```python
from build123d import *

# Parameters (mm, degrees)
EXTRUDE_1_DEPTH              = 10
SKETCH_2_W                   = 43
SKETCH_2_H                   = 10
EXTRUDE_2_DEPTH              = 24.24999999999997
EXTRUDE_3_DEPTH              = 6.6999999999999975
CUT_EXTRUDE_START            = -1.449999999999993
CUT_EXTRUDE_1_DEPTH          = 1.449999999999993
EXTRUDE_4_DEPTH              = 16.349999999999994
SKETCH_6_W                   = 35.2
SKETCH_6_H                   = 8.099999999999994
CUT_EXTRUDE_2_DEPTH          = 5
SKETCH_7_W                   = 9.999999999999998
SKETCH_7_H                   = 8.7
EXTRUDE_5_DEPTH              = 8.999999999999995
HOLE_WIZARD_3_3_3_3_1_D      = 3.3
HOLE_WIZARD_3_3_3_3_1_DEPTH  = 8.5
HOLE_WIZARD_3_3_3_3_1_TIP    = 0.9914200213954745
HOLE_WIZARD_3_3_3_3_2_D      = 3.3
HOLE_WIZARD_3_3_3_3_2_DEPTH  = 8.5
HOLE_WIZARD_3_3_3_3_2_TIP    = 0.9914200213954745
HOLE_WIZARD_3_3_3_3_3_D      = 3.3
HOLE_WIZARD_3_3_3_3_3_DEPTH  = 9
HOLE_WIZARD_3_3_3_3_3_TIP    = 0.9914200213954745
HOLE_WIZARD_15_0_15_1_D      = 15
HOLE_WIZARD_15_0_15_1_DEPTH  = 24.25
HOLE_WIZARD_M3_1_D           = 3.4
HOLE_WIZARD_M3_1_DEPTH       = 16.7
HOLE_WIZARD_M3_1_CBORE_D     = 6.5
HOLE_WIZARD_M3_1_CBORE_DEPTH = 4.75
HOLE_WIZARD_4_0_4_1_D        = 4
HOLE_WIZARD_4_0_4_1_DEPTH    = 16.7
FILLET_1_R                   = 0.5
CHAMFER_1_SIZE               = 0.4999999999999948
FILLET_2_R                   = 2


with BuildPart() as part:
    # 草图1 → 凸台-拉伸1 (new body)
    with BuildSketch(Plane(origin=(0, -51, 0), x_dir=(1, 0, 0), z_dir=(0, 1, 0))):
        with BuildLine():
            Line((21.5, -35.60000000000002), (-21.5, -35.59999999999997))
            ThreePointArc((-21.5, -35.59999999999997), (-20.657569635687853, -36.07468782040316), (-20.1362960848869, -36.8891148157745))
            ThreePointArc((-20.1362960848869, -36.8891148157745), (-3.42e-15, -51.35000000000001), (20.1362960848869, -36.8891148157745))
            ThreePointArc((20.1362960848869, -36.8891148157745), (20.65756963568787, -36.07468782040319), (21.5, -35.60000000000002))
        make_face()
    extrude(amount=-EXTRUDE_1_DEPTH)

    # 草图2 → 凸台-拉伸2 (add)
    with BuildSketch(Plane(origin=(-4.021e-14, 0, 35.599999999999994), x_dir=(-1, 0, -1.13e-15), z_dir=(1.13e-15, 0, -1))):
        with Locations((-4.086e-14, -56.00000000000001)):
            Rectangle(SKETCH_2_W, SKETCH_2_H)
    extrude(amount=EXTRUDE_2_DEPTH)

    # 草图3 → 凸台-拉伸3 (add)
    with BuildSketch(Plane.XZ.offset(61)):
        with BuildLine():
            Line((-4.85285709567227, 48.211109242919996), (-5.499904708428581, 50.625923808642696))
            ThreePointArc((-5.499904708428581, 50.625923808642696), (1.3e-15, 51.349999999999994), (5.499904708428581, 50.625923808642696))
            Line((5.499904708428581, 50.625923808642696), (4.852857095672274, 48.21110924292003))
            ThreePointArc((4.852857095672274, 48.21110924292003), (5.799211712715089, 46.409565616324066), (7.6704851839498795, 47.209241860550264))
            ThreePointArc((7.6704851839498795, 47.209241860550264), (-3.02e-15, 11.349999999999994), (-7.67048518394987, 47.209241860550264))
            ThreePointArc((-7.67048518394987, 47.209241860550264), (-5.799211712715104, 46.40956561632406), (-4.85285709567227, 48.211109242919996))
        make_face()
    extrude(amount=EXTRUDE_3_DEPTH)

    # 草图4 → 切除-拉伸1 (cut)
    with BuildSketch(Plane.XZ.offset(67.7).offset(CUT_EXTRUDE_START)):
        with BuildLine():
            ThreePointArc((7.6704851839498795, 47.209241860550264), (5.799211712715057, 46.409565616324066), (4.85285709567228, 48.211109242920095))
            ThreePointArc((4.85285709567228, 48.211109242920095), (-7.18e-15, 48.850000000000065), (-4.85285709567227, 48.211109242919996))
            ThreePointArc((-4.85285709567227, 48.211109242919996), (-5.799211712715106, 46.409565616324066), (-7.67048518394987, 47.209241860550264))
            ThreePointArc((-7.67048518394987, 47.209241860550264), (-3.44e-15, 11.349999999999998), (7.6704851839498795, 47.209241860550264))
        make_face()
    extrude(amount=CUT_EXTRUDE_1_DEPTH, mode=Mode.SUBTRACT)

    # 草图5 → 凸台-拉伸4 (add)
    with BuildSketch(Plane(origin=(-1.282e-14, 0, 11.35000000000002), x_dir=(-1, 0, -1.13e-15), z_dir=(1.13e-15, 0, -1))):
        Polygon((21.499999999999986, -51), (21.499999999999986, -61), (-21.500000000000007, -61), (-21.50000000000001, -51), align=None)
    extrude(amount=EXTRUDE_4_DEPTH)

    # 草图6 → 切除-拉伸2 (cut)
    with BuildSketch(Plane(origin=(5.65e-15, 0, -4.999999999999973), x_dir=(-1, 0, -1.13e-15), z_dir=(1.13e-15, 0, -1))):
        with Locations((7.11e-15, -55.050000000000004)):
            Rectangle(SKETCH_6_W, SKETCH_6_H)
    extrude(amount=-CUT_EXTRUDE_2_DEPTH, mode=Mode.SUBTRACT)

    # 草图7 → 凸台-拉伸5 (add)
    with BuildSketch(Plane(origin=(0, -51, 0), x_dir=(-1, 0, 0), z_dir=(0, 1, 0))):
        with Locations((-8.9e-16, 4.35)):
            Rectangle(SKETCH_7_W, SKETCH_7_H)
    extrude(amount=EXTRUDE_5_DEPTH)

    # Ø3.3 (3.3) 直径孔1
    with Locations(Plane(origin=(21.50000000000004, 0, 2.429e-14), x_dir=(1.13e-15, 0, -1), z_dir=(1, 0, 1.13e-15))):
        with Locations((-15.1, -56), (-30.1, -56)):
            Hole(HOLE_WIZARD_3_3_3_3_1_D / 2, depth=HOLE_WIZARD_3_3_3_3_1_DEPTH)
            with Locations((0, 0, -(HOLE_WIZARD_3_3_3_3_1_DEPTH + HOLE_WIZARD_3_3_3_3_1_TIP / 2))):  # 118° drill point
                Cone(0, HOLE_WIZARD_3_3_3_3_1_D / 2, HOLE_WIZARD_3_3_3_3_1_TIP, mode=Mode.SUBTRACT)

    # Ø3.3 (3.3) 直径孔2
    with Locations(Plane.ZY.offset(21.499999999999957)):
        with Locations((15.1, -56), (30.1, -56)):
            Hole(HOLE_WIZARD_3_3_3_3_2_D / 2, depth=HOLE_WIZARD_3_3_3_3_2_DEPTH)
            with Locations((0, 0, -(HOLE_WIZARD_3_3_3_3_2_DEPTH + HOLE_WIZARD_3_3_3_3_2_TIP / 2))):  # 118° drill point
                Cone(0, HOLE_WIZARD_3_3_3_3_2_D / 2, HOLE_WIZARD_3_3_3_3_2_TIP, mode=Mode.SUBTRACT)

    # Ø3.3 (3.3) 直径孔3
    with Locations(Plane(origin=(0, 0, 0), x_dir=(-1, 0, -1.13e-15), z_dir=(1.13e-15, 0, -1))):
        with Locations((-9.5, -55), (9.5, -55)):
            Hole(HOLE_WIZARD_3_3_3_3_3_D / 2, depth=HOLE_WIZARD_3_3_3_3_3_DEPTH)
            with Locations((0, 0, -(HOLE_WIZARD_3_3_3_3_3_DEPTH + HOLE_WIZARD_3_3_3_3_3_TIP / 2))):  # 118° drill point
                Cone(0, HOLE_WIZARD_3_3_3_3_3_D / 2, HOLE_WIZARD_3_3_3_3_3_TIP, mode=Mode.SUBTRACT)

    # Ø15.0 (15) 直径孔1
    with Locations(Plane.XZ.offset(66.25)):
        with Locations((0, 30.1)):
            Hole(HOLE_WIZARD_15_0_15_1_D / 2, depth=HOLE_WIZARD_15_0_15_1_DEPTH)

    # M3 六角头机械螺钉的柱形沉头孔1
    with Locations(Plane(origin=(0, -51, 0), x_dir=(1, 0, 0), z_dir=(0, 1, 0))):
        with Locations((0, -43.6), (-11.691342951, -36.85), (-11.691342951, -23.35), (0, -16.6), (11.691342951, -23.35), (11.691342951, -36.85)):
            CounterBoreHole(HOLE_WIZARD_M3_1_D / 2, HOLE_WIZARD_M3_1_CBORE_D / 2, HOLE_WIZARD_M3_1_CBORE_DEPTH, depth=HOLE_WIZARD_M3_1_DEPTH)

    # Ø4.0 (4) 直径孔1
    with Locations(Plane(origin=(0, -51, 0), x_dir=(1, 0, 0), z_dir=(0, 1, 0))):
        with Locations((21.5, 5), (-21.5, 5)):
            Hole(HOLE_WIZARD_4_0_4_1_D / 2, depth=HOLE_WIZARD_4_0_4_1_DEPTH)

    # 圆角1
    fillet_1_edges = [part.edges().sort_by_distance(p)[0] for p in [
        (-21.499999999999954, -56, -3),
        (-19.5, -56, -4.9999999999999964),
        (19.5, -56, -4.999999999999999),
        (21.500000000000043, -56, -3),
        (-4.852857095672272, -66.97500000000001, 48.211109242919996),
        (4.852857095672273, -66.97500000000001, 48.21110924292003),
        (5.499904708428581, -64.35, 50.625923808642696),
        (-5.499904708428581, -64.35, 50.625923808642696),
        (7.6704851839498795, -63.62500000000001, 47.209241860550264),
        (-7.670485183949873, -63.62500000000001, 47.209241860550264),
        (-21.5, -56, 35.59999999999997),
        (21.5, -56, 35.60000000000002),
        (-4.999999999999998, -46.5, 8.7),
        (5, -46.5, 8.7),
    ]]
    fillet(fillet_1_edges, radius=FILLET_1_R)

    # 倒角1
    chamfer_1_edges = [part.edges().sort_by_distance(p)[0] for p in [
        (5, -42.00000000000001, 4.1),
        (8.9e-16, -42.00000000000001, 8.7),
        (-4.853553390593272, -42.00000000000001, 8.553553390593272),
        (4.853553390593274, -42.00000000000001, 8.553553390593272),
        (-4.999999999999998, -42.00000000000001, 4.1),
    ]]
    chamfer(chamfer_1_edges, length=CHAMFER_1_SIZE)

    # 圆角2
    fillet_2_edges = [part.edges().sort_by_distance(p)[0] for p in [
        (-17.600000000000005, -59.1, -2.499999999999993),
        (17.599999999999998, -59.1, -2.499999999999954),
    ]]
    fillet(fillet_2_edges, radius=FILLET_2_R)


solid = part.part
```
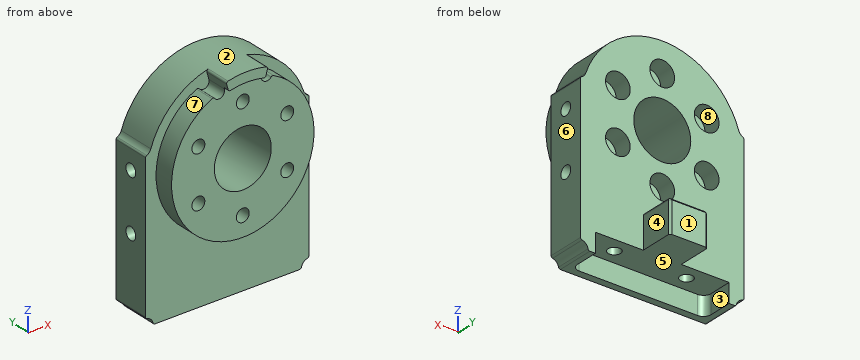
For this review, take the finished solid that the model builds, in its own axes (mm). Face numbers are marked on the shaded views. A direction names the side the tool comes from. Round coordinates to 2 decimals unless told otherwise and drop trailing zeros. Write each loop counter-clockwise with the first axis right and the second up, starting at its lowest first coordinate (ties: lowest second). Pieces come first, ordered by that corner, then holes. Notation, with made-up numbers: (72, 41.25) -> (84, 41.25) arc R25 cw to (84, 68.25) -> close; hole circle Ø9 at (-10, -6.75). An arc over 180 degrees is marked (long way). Use one line per item in the form item = value.
Q1. Consider section D-D (y = -46.5). State the section outline as (x, z) points.
Resolved:
outline = (-5, 0) -> (5, 0) -> (5, 8.2) arc R0.5 ccw to (4.5, 8.7) -> (-4.5, 8.7) arc R0.5 ccw to (-5, 8.2) -> close
Q2. To check wall thickness, follow probe 1 along X at (y, z) = (-55, 7); probe 2 along Z at (x, y) = (0, -60.5); probe 3 along Y at (x, z) = (19.5, 30.1). State the ranges of each line that lie inside material, in increasing order. Write a range as from..to.
Resolved:
probe_1 = -21.5..-11.15, -7.85..7.85, 11.15..21.5
probe_2 = -5..14.9, 18.3..22.6, 37.6..41.9, 45.3..51.35
probe_3 = -61..-57.65, -54.35..-51
Q3. Machinability: for the marked faces 4, 5, 6, 7 and 8, which of the approach directions +Z, -Z, +X, -X, +Y, -Y give a long, thin tool a straight path to every point of the face, cutting with its end or side? Answer none if there is none.
Resolved:
face_4 = +Z, -Z, +X, +Y
face_5 = -Z, +Y
face_6 = +Z, -Z, +X, +Y, -Y
face_7 = -Y
face_8 = +Y
Q4. The part is to be moulded in two halves that separate along X. For the marked faces 1, 2 and 3, say which applies: released by +X, released by -X, zero draft, split by the parting line, or undercut.
Resolved:
face_1 = zero draft
face_2 = split by the parting line
face_3 = undercut
Q5. Clearance check with flat-ended pins moving along their axes: pin 1 Ø10 at (x, z) = (-15, 5.5) entering from +Y; pin 2 Ø2 at (x, z) = (-0.5, 35.5) entering from -Y; pin 3 Ø9.5 at (x, y) = (0.5, -48.5) entering from +Z; pin 4 Ø2.5 at (y, z) = (-46.5, 3) entering from -X. State where each tip first meets the part, or that it passes through.
Resolved:
pin_1 = -51
pin_2 = through
pin_3 = 51.35
pin_4 = -5
Q6. Consider section A-A (z = 5.5). State the section outline as (x, y) points.
Resolved:
outline = (-21.5, -61) -> (21.5, -61) -> (21.5, -51) -> (5, -51) -> (5, -42.5) -> (4.5, -42) -> (-4.5, -42) -> (-5, -42.5) -> (-5, -51) -> (-21.5, -51) -> close; hole circle Ø3.3 at (-9.5, -55); hole circle Ø3.3 at (9.5, -55)
Q7. Consider section B-B (z = 43.6). State the section outline as (x, y) points, then the cut area to 3 significant figures.
Resolved:
outline = (-16.41, -61) -> (-13.01, -61) -> (-13.01, -66.25) -> (-1.7, -66.25) -> (-1.7, -55.75) -> (-3.25, -55.75) -> (-3.25, -51) -> (-16.41, -51) -> close; (1.7, -66.25) -> (13.01, -66.25) -> (13.01, -61) -> (16.41, -61) -> (16.41, -51) -> (3.25, -51) -> (3.25, -55.75) -> (1.7, -55.75) -> close
area = 398 mm²
Q8. Consider section C-C (y = -52). State the section outline as (x, z) points, then the cut area to 3 significant figures.
Resolved:
outline = (-21.5, -2.55) arc R0.5 ccw to (-21.1, -3.04) arc R2 cw to (-19.54, -4.6) arc R0.5 ccw to (-19.05, -5) -> (-17.6, -5) -> (-17.6, 0) -> (17.6, 0) -> (17.6, -5) -> (19.05, -5) arc R0.5 ccw to (19.54, -4.6) arc R2 cw to (21.1, -3.04) arc R0.5 ccw to (21.5, -2.55) -> (21.5, 35.25) arc R0.5 ccw to (21.21, 35.71) arc R2 cw to (20.14, 36.89) arc R21.25 ccw to (-20.14, 36.89) arc R2 cw to (-21.21, 35.71) arc R0.5 ccw to (-21.5, 35.25) -> close; hole circle Ø6.5 at (-11.69, 23.35); hole circle Ø6.5 at (-11.69, 36.85); hole circle Ø15 at (0, 30.1); hole circle Ø6.5 at (0, 16.6); hole circle Ø6.5 at (0, 43.6); hole circle Ø6.5 at (11.69, 23.35); hole circle Ø6.5 at (11.69, 36.85)
area = 1,670 mm²
